```python
from build123d import *

# Parameters (mm, degrees)
SKETCH1_W           = 60
SKETCH1_H           = 43.5
SKETCH1_R           = 1.5
SKETCH1_W_2         = 23
SKETCH1_H_2         = 12
SKETCH1_W_3         = 15
SKETCH1_H_3         = 3
SKETCH1_W_4         = 10
SKETCH1_W_5         = 3
SKETCH1_H_4         = 6
SKETCH1_H_5         = 4
BOSS_EXTRUDE1_DEPTH = 2.75
FILLET1_R           = 4


with BuildPart() as part:
    # Sketch1 → Boss-Extrude1 (new body)
    with BuildSketch(Plane.XY):
        with Locations((-7.382405678, -3.098084383)):
            Rectangle(SKETCH1_W, SKETCH1_H)
        with Locations((-17.369283231, -22.348084383)):
            Circle(SKETCH1_R, mode=Mode.SUBTRACT)
        with Locations((-17.369283231, -4.348084383)):
            Circle(SKETCH1_R, mode=Mode.SUBTRACT)
        with Locations((18.630716769, 8.151915617)):
            Circle(SKETCH1_R, mode=Mode.SUBTRACT)
        with Locations(Location((-33.395528126, 8.151915617, 0), (0, 0, 180))):
            Circle(SKETCH1_R, mode=Mode.SUBTRACT)
        with Locations((-17.382405678, -13.348084383)):
            Rectangle(SKETCH1_W_2, SKETCH1_H_2, mode=Mode.SUBTRACT)
        with Locations((-22.882405678, 12.151915617)):
            Rectangle(SKETCH1_W_3, SKETCH1_H_3, mode=Mode.SUBTRACT)
        with Locations((9.617594322, 12.191282959)):
            Rectangle(SKETCH1_W_4, SKETCH1_H_3, mode=Mode.SUBTRACT)
        with Locations((18.617594322, 1.151915617)):
            Rectangle(SKETCH1_W_5, SKETCH1_H_4, mode=Mode.SUBTRACT)
        with Locations((18.617594322, 15.151915617)):
            Rectangle(SKETCH1_W_5, SKETCH1_H_5, mode=Mode.SUBTRACT)
        Polygon((-31.882405678, 4.151915617), (-34.882405678, 4.151915617), (-34.882405678, 1.688906326), (-31.8745626, 1.688906326), align=None, mode=Mode.SUBTRACT)
        Polygon((-34.882405678, -1.848084383), (-34.882405678, 0.693659593), (-31.8745626, 0.693659593), (-31.882405678, -1.848084383), align=None, mode=Mode.SUBTRACT)
        with Locations((-33.382405678, 15.151915617)):
            Rectangle(SKETCH1_W_5, SKETCH1_H_5, mode=Mode.SUBTRACT)
    extrude(amount=BOSS_EXTRUDE1_DEPTH)

    # Fillet1
    fillet1_edges = [part.edges().sort_by_distance(p)[0] for p in [
        (22.617594322, -24.848084383, 1.375),
        (-37.382405678, -24.848084383, 1.375),
        (-37.382405678, 18.651915617, 1.375),
        (22.617594322, 18.651915617, 1.375),
    ]]
    fillet(fillet1_edges, radius=FILLET1_R)


solid = part.part
```
Verification items for the finished model (mm, model axes). A direction names the side the tool comes from. Coordinates: 2 decimals unless noted, no trailing zeros. Order: outer loops, then holes, each group sorted by start corner. A loop starts at its lowest first (then second) coordinate and runs counter-clockwise, first axis right, second up. Notation, with made-up numbers: (0.25, -20) -> (46.25, -20) arc R22 ccw to (46.25, 16) -> close; hole circle Ø9 at (-23, -21.75). An arc over 180 degrees is marked (long way). Put each result on its own line as item: value. Start each with the question number.
1) Tool access check on faces 1 (the flat face through (22.618, -3, 1)), 2 (the flat face through (10, 13.691, 1)). Record the directions out of +Z, -Z, +X, -X, +Y, -Y that give a thin tool (end or side, any length) a straight path to the whole face; none if there is none.
2) Cross-section at C-C (y = -17.5). Enter the section's corners in (x, z), plus the area to 3 significant figures.
3) Cross-section at B-B (x = -26). Enter the section's corners in (y, z), plus the area to 3 significant figures.
4) Cross-section at D-D (y = -1). Enter the section's corners in (x, z), plus the area to 3 significant figures.
5) Material ranges on L1, parallel to Y at x = -25.5, z = 2.25; L2, parallel to X at y = 0.5, z = 2.5; L3, parallel to X at y = -16, z = 0.35, recorded low to high.
6) Cross-section at A-A (x = -12.5). Enter the section's corners in (y, z), plus the area to 3 significant figures.
7) Go/stop test with a flat-tipped pin: pin 1 (12 mm diameter, centred on x = 7.5, y = 6.5, fed in from -Z). Record where the tip stops, or that it passes through.
8) Release check for a two-part mould opening along X. For faces 3 (the flat face through (-37.382, -3, 1)), 4 (the flat face through (-8, 18.652, 1)), 5 (the flat face through (17.118, 1, 1)) record: pulls with the +X half, pulls with the -X half, needs draft (parallel to the pull), parting line crosses it, or undercut.
Geometry check:
1. face 1: +Z, -Z, +X, +Y, -Y
1. face 2: +Z, -Z
2. outline: (-37.38, 0) -> (-28.88, 0) -> (-28.88, 2.75) -> (-37.38, 2.75) -> close; (-5.88, 0) -> (22.62, 0) -> (22.62, 2.75) -> (-5.88, 2.75) -> close
2. area: 102 mm^2
3. outline: (-24.85, 0) -> (-19.35, 0) -> (-19.35, 2.75) -> (-24.85, 2.75) -> close; (-7.35, 0) -> (10.65, 0) -> (10.65, 2.75) -> (-7.35, 2.75) -> close; (13.65, 0) -> (18.65, 0) -> (18.65, 2.75) -> (13.65, 2.75) -> close
3. area: 78.4 mm^2
4. outline: (-37.38, 0) -> (-34.88, 0) -> (-34.88, 2.75) -> (-37.38, 2.75) -> close; (-31.88, 0) -> (17.12, 0) -> (17.12, 2.75) -> (-31.88, 2.75) -> close; (20.12, 0) -> (22.62, 0) -> (22.62, 2.75) -> (20.12, 2.75) -> close
4. area: 148 mm^2
5. L1: y = -24.85 to -19.35, -7.35 to 10.65, 13.65 to 18.65
5. L2: x = -37.38 to -34.88, -31.88 to 17.12, 20.12 to 22.62
5. L3: x = -37.38 to -28.88, -5.88 to 22.62
6. outline: (-24.85, 0) -> (-19.35, 0) -> (-19.35, 2.75) -> (-24.85, 2.75) -> close; (-7.35, 0) -> (18.65, 0) -> (18.65, 2.75) -> (-7.35, 2.75) -> close
6. area: 86.6 mm^2
7. pin 1: stops at z = 0
8. face 3: pulls with the -X half
8. face 4: needs draft
8. face 5: undercut
